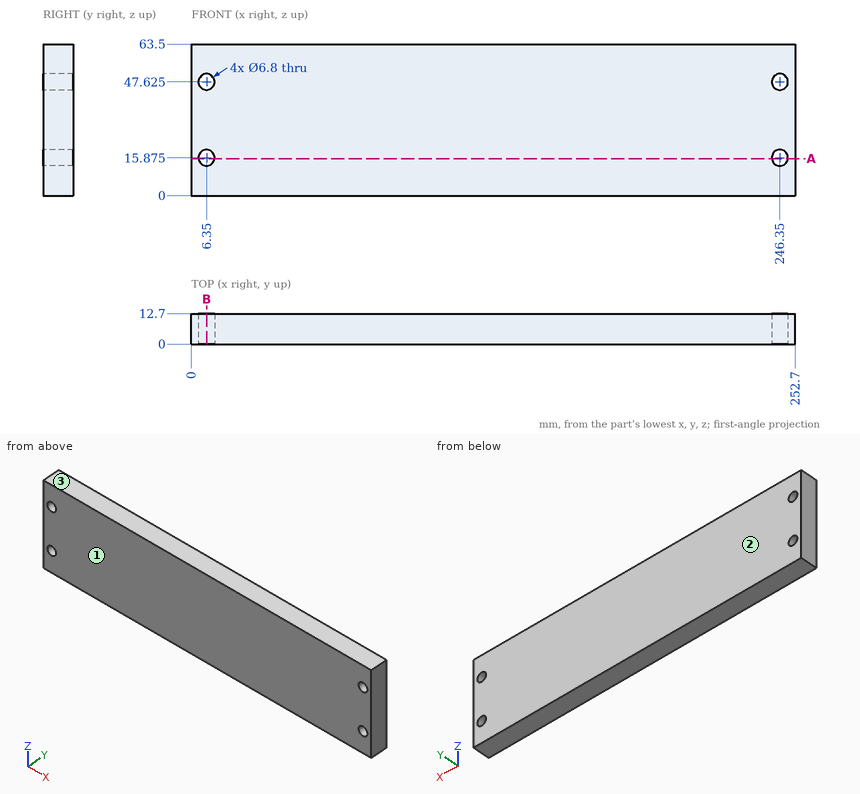
Drawing for the job (mm, zero at the part's lowest x, y, z). Round coordinates to 2 decimals unless told otherwise and drop trailing zeros. Write each loop counter-clockwise with the first axis right and the second up, starting at its lowest first coordinate (ties: lowest second). Pieces come first, ordered by that corner, then holes. Notation, with made-up numbers: M -36,-8.75 L 22,-8.75 A21 ccw 22,26.25 Z; hole C 19.5,45.5 d3. An arc over 180 degrees is marked long. Answer as a JSON object with one key per item and string values. Group by question number.
(1) Drill centre lines: L1, parallel to X at y = 4.5, z = 47.5; L2, parallel to Z at x = 246.35, y = 8.75 (3 decimals); L3, parallel to X at y = 8.75, z = 18. Where is each one in solid material? Low to high.
(2) Cut at A-A (z = 15.5). Give the cut face in (x, y).
(3) Mould opens along Y. For the marked faces 1, 2 and 3 say: pulls with the +Y half, pulls with the -Y half, needs draft (parallel to the pull), parting line crosses it, or undercut.
(4) Cut at B-B (x = 6.35). Give the cut face in (y, z) (3 decimals), and give its area (3 significant figures).
Responses:
{
 "1": {"L1": "x = 0 to 2.95, 9.75 to 242.95, 249.75 to 252.7", "L2": "z = 0 to 12.475, 19.275 to 44.225, 51.025 to 63.5", "L3": "x = 0 to 3.7, 9 to 243.7, 249 to 252.7"},
 "2": {"outline": "M 0,0 L 2.97,0 L 2.97,12.7 L 0,12.7 Z; M 9.73,0 L 242.97,0 L 242.97,12.7 L 9.73,12.7 Z; M 249.73,0 L 252.7,0 L 252.7,12.7 L 249.73,12.7 Z"},
 "3": {"face 1": "pulls with the -Y half", "face 2": "pulls with the +Y half", "face 3": "needs draft"},
 "4": {"outline": "M 0,0 L 12.7,0 L 12.7,12.475 L 0,12.475 Z; M 0,19.275 L 12.7,19.275 L 12.7,44.225 L 0,44.225 Z; M 0,51.025 L 12.7,51.025 L 12.7,63.5 L 0,63.5 Z", "area": "634 mm2"}
}
